from build123d import *

# Parameters (mm, degrees)
SKICA1_W                 = 120
SKICA1_H                 = 80
P_IDAT_VYSUNUT_M1_DEPTH  = 12
SKICA2_R                 = 5
ODEBRAT_VYSUNUT_M1_DEPTH = 12
LINPOLE1_COUNT           = 7
LINPOLE1_PITCH           = 15
LINPOLE1_COUNT_DIR2      = 5
LINPOLE1_PITCH_DIR2      = 15


with BuildPart() as part:
    # Skica1 → Přidat vysunutím1 (new body)
    with BuildSketch(Plane.XY):
        Rectangle(SKICA1_W, SKICA1_H)
    extrude(amount=P_IDAT_VYSUNUT_M1_DEPTH)

    # Skica2 → Odebrat vysunutím1 (cut)
    with BuildSketch(Plane(origin=(0, 0, 0), x_dir=(-1, 0, 0), z_dir=(0, 0, -1))):
        with Locations((-45, -30)):
            Circle(SKICA2_R)
    odebrat_vysunut_m1 = extrude(amount=-ODEBRAT_VYSUNUT_M1_DEPTH, mode=Mode.SUBTRACT)

    # LinPole1: Odebrat vysunut_m1 7 × 5, 9 skipped
    with Locations(*[(-i * LINPOLE1_PITCH, j * LINPOLE1_PITCH_DIR2, 0) for i in range(LINPOLE1_COUNT) for j in range(LINPOLE1_COUNT_DIR2) if (i, j) not in ((0, 0), (1, 0), (1, 4), (2, 1), (2, 3), (3, 2), (4, 1), (4, 3), (5, 0), (5, 4))]):
        add(odebrat_vysunut_m1, mode=Mode.SUBTRACT)


solid = part.part
The listing builds one solid part. Answer for the finished solid, in the listing's coordinates (mm). Give positions to 0.01 mm unless a question says otherwise; leave off trailing zeros. Loops run counter-clockwise (first coordinate to the right, second up) from the corner with the lowest first, then second, coordinate; pieces in that order, holes last.
Item 1: Determine the mould class of faces 1 (the flat face through (-1, 40, 6)), 2 (the cylindrical face through (-41, -33, 6)), 3 (the cylindrical face through (1.08, -19.88, 5.92)), 4 (the flat face through (-1, -40, 6)) for opening direction Y: +Y half, -Y half, draft (parallel to the pull), parting line (faces both ways), or undercut.
Derived:
face 1: +Y half
face 2: undercut
face 3: undercut
face 4: -Y half
Item 2: A cutting plane is placed at B-B (y = 0). Give the vertices of the cut face in (x, z), then the cut area to 3 significant figures.
Derived:
outline: (-60, 0) - (-50, 0) - (-50, 12) - (-60, 12) - close; (-40, 0) - (-35, 0) - (-35, 12) - (-40, 12) - close; (-25, 0) - (-20, 0) - (-20, 12) - (-25, 12) - close; (-10, 0) - (10, 0) - (10, 12) - (-10, 12) - close; (20, 0) - (25, 0) - (25, 12) - (20, 12) - close; (35, 0) - (40, 0) - (40, 12) - (35, 12) - close; (50, 0) - (60, 0) - (60, 12) - (50, 12) - close
area: 720 mm2
Item 3: A cutting plane is placed at C-C (x = 0). Give the vertices of the cut face in (y, z).
Derived:
outline: (-40, 0) - (-35, 0) - (-35, 12) - (-40, 12) - close; (-25, 0) - (-20, 0) - (-20, 12) - (-25, 12) - close; (-10, 0) - (10, 0) - (10, 12) - (-10, 12) - close; (20, 0) - (25, 0) - (25, 12) - (20, 12) - close; (35, 0) - (40, 0) - (40, 12) - (35, 12) - close
Item 4: A cutting plane is placed at A-A (x = 15). Give the vertices of the cut face in (y, z), then the cut area to 3 significant figures.
Derived:
outline: (-40, 0) - (-35, 0) - (-35, 12) - (-40, 12) - close; (-25, 0) - (-5, 0) - (-5, 12) - (-25, 12) - close; (5, 0) - (25, 0) - (25, 12) - (5, 12) - close; (35, 0) - (40, 0) - (40, 12) - (35, 12) - close
area: 600 mm2
Item 5: Each of these flat-tipped pins is pushed along its axis until it touches: pin 1 Ø13 at (x, y) = (-45, 15) entering from +Z; pin 2 Ø9 at (x, y) = (15, 30) entering from -Z. Where does it stop, or does it pass through?
Derived:
pin 1: stops at z = 12
pin 2: passes through
Item 6: Find the intervals of material crossed by line 1 along Y through (x, z) = (-45, 5.5); line 2 along Y through (x, z) = (30, 6.75); line 3 along Y through (x, z) = (0, 3), in increasing order.
Derived:
line 1: y = -40 to -35, -25 to -20, -10 to -5, 5 to 10, 20 to 25, 35 to 40
line 2: y = -40 to -20, -10 to -5, 5 to 10, 20 to 40
line 3: y = -40 to -35, -25 to -20, -10 to 10, 20 to 25, 35 to 40
Item 7: A cutting plane is placed at D-D (z = 6.25). Give the number of separate pieces and of enclosed holes in the cut face, then the cut area to 3 significant figures.
Derived:
separate pieces: 1
enclosed holes: 26
area: 7,560 mm2
